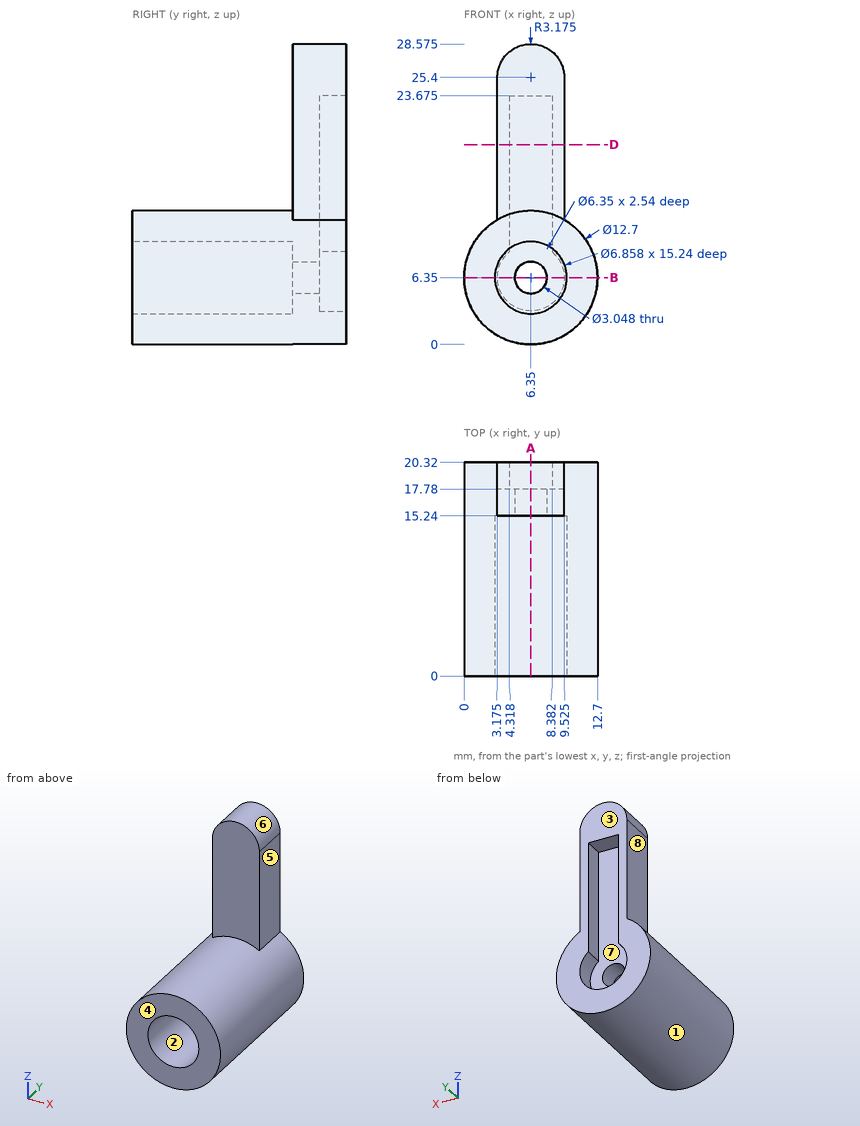
Study the drawing (mm; zero at the part's minimum x, y, z) and answer. A direction names the side the tool comes from. Give positions to 0.01 mm unless a question says otherwise; leave off trailing zeros. Loops run counter-clockwise (first coordinate to the right, second up) from the corner with the lowest first, then second, coordinate; pieces in that order, holes last. Notation, with made-up numbers: (-36.75, 64) - (0.25, 64) arc R4 cw to (0.25, 69) - close; hole circle Ø11 at (33.25, 89). An arc over 180 degrees is marked (long way). Use CSV: the item, a comma, the result in double quotes. Start each with the question number.
(1) Each of these flat-tipped pins is pushed along its axis until it touches: pin 1 (1.3 mm diameter, centred on y = 19, z = 16, fed in from +X) (3 decimals); pin 2 (3.5 mm diameter, centred on x = 7.5, z = 6, fed in from -Y); pin 3 (1.5 mm diameter, centred on y = 17, z = 17, fed in from -X) (3 decimals); pin 4 (2 mm diameter, centred on y = 11.5, z = 7.5, fed in from -X). Where does it stop, or does it pass through?
(2) Determine the mould class of the marked faces 1, 2 and 3 for opening direction Z: released by +Z, released by -Z, zero draft, split by the parting line, or undercut.
(3) Find section A-A, the plane x = 6.35. Determine the outline of the cut face in (y, z) (1 decimal).
(4) Find the intervals of material crossed by L1, parallel to X at y = 17, z = 6.35; L2, parallel to X at y = 18.5, z = 19.5 (1 decimal); L3, parallel to Y at x = 5.25, z = 18.25, in increasing order.
(5) Find section D-D, the plane z = 19. Determine the outline of the cut face in (x, y) (1 decimal).
(6) A tool of negligible diameter and unlimited length cuts with its end or side. For the marked faces 4, 5, 6, 7 and 8, from which of +Z, -Z, +X, -X, +Y, -Y can it reach the whole face along a straight path? Write none if from no direction.
(7) Find section B-B, the plane z = 6.35. Determine the outline of the cut face in (x, y) (1 decimal), plus the area to 3 significant figures.
Results found:
1,pin 1,"x = 9.525"
1,pin 2,"y = 15.24"
1,pin 3,"x = 3.175"
1,pin 4,"x = 0"
2,face 1,"split by the parting line"
2,face 2,"undercut"
2,face 3,"zero draft"
3,outline,"(0, 0) - (20.3, 0) - (20.3, 3.2) - (17.8, 3.2) - (17.8, 4.8) - (15.2, 4.8) - (15.2, 2.9) - (0, 2.9) - close; (0, 9.8) - (15.2, 9.8) - (15.2, 7.9) - (17.8, 7.9) - (17.8, 23.7) - (20.3, 23.7) - (20.3, 28.6) - (15.2, 28.6) - (15.2, 12.7) - (0, 12.7) - close"
4,L1,"0 to 4.83, 7.87 to 12.7"
4,L2,"3.2 to 4.3, 8.4 to 9.5"
4,L3,"15.24 to 17.78"
5,outline,"(3.2, 15.2) - (9.5, 15.2) - (9.5, 20.3) - (8.4, 20.3) - (8.4, 17.8) - (4.3, 17.8) - (4.3, 20.3) - (3.2, 20.3) - close"
6,face 4,"+Z, -Z, +X, -X, -Y"
6,face 5,"+Z, +X, +Y, -Y"
6,face 6,"+Z, +Y, -Y"
6,face 7,"+Y"
6,face 8,"+Z, -X, +Y, -Y"
7,outline,"(0, 0) - (2.9, 0) - (2.9, 15.2) - (4.8, 15.2) - (4.8, 17.8) - (3.2, 17.8) - (3.2, 20.3) - (0, 20.3) - close; (7.9, 15.2) - (9.8, 15.2) - (9.8, 0) - (12.7, 0) - (12.7, 20.3) - (9.5, 20.3) - (9.5, 17.8) - (7.9, 17.8) - close"
7,area,"130 mm^2"
